```python
from build123d import *

# Parameters (mm, degrees)
SKETCH1_R           = 1.25
BOSS_EXTRUDE1_DEPTH = 0.1


with BuildPart() as part:
    # Sketch1 → Boss-Extrude1 (new body)
    with BuildSketch(Plane(origin=(0, 0, 0), x_dir=(1, 0, 0), z_dir=(0, 1, 0))):
        with BuildLine():
            Line((-34.25, 1.4), (-18.774596669, 1.4))
            ThreePointArc((-18.774596669, 1.4), (-18, 1.6), (-17.225403331, 1.4))
            Line((-17.225403331, 1.4), (17.225403331, 1.4))
            ThreePointArc((17.225403331, 1.4), (18, 1.6), (18.774596669, 1.4))
            Line((18.774596669, 1.4), (34.25, 1.4))
            Line((34.25, 1.4), (34.25, -1.4))
            Line((34.25, -1.4), (18.774596669, -1.4))
            ThreePointArc((18.774596669, -1.4), (18, -1.6), (17.225403331, -1.4))
            Line((17.225403331, -1.4), (-17.225403331, -1.4))
            ThreePointArc((-17.225403331, -1.4), (-18, -1.6), (-18.774596669, -1.4))
            Line((-18.774596669, -1.4), (-34.25, -1.4))
            Line((-34.25, -1.4), (-34.25, 1.4))
        make_face()
        with Locations(Location((-18, 0, 0), (0, 0, 270))):
            Circle(SKETCH1_R, mode=Mode.SUBTRACT)
        with Locations(Location((18, 0, 0), (0, 0, 90))):
            Circle(SKETCH1_R, mode=Mode.SUBTRACT)
    extrude(amount=BOSS_EXTRUDE1_DEPTH)


solid = part.part
```
Part model, mm, in its own coordinate system. Round coordinates to 2 decimals unless told otherwise and drop trailing zeros. Loops run counter-clockwise (first coordinate to the right, second up) from the corner with the lowest first, then second, coordinate; pieces in that order, holes last.
Item 1: Cut at B-B, the plane x = 18. Give the cut face in (y, z), then the cut area to 3 significant figures.
Item 2: Drill centre lines: line 1 (X direction, y = 0.05, z = 0); line 2 (Z direction, x = 18, y = 0.05); line 3 (Z direction, x = 25.5, y = 0.05). Where is each one in solid material? Low to high.
Item 3: Cut at A-A, the plane z = 0. Give the cut face in (x, y).
Item 4: Cut at C-C, the plane x = 7.5. Give the cut face in (y, z), then the cut area to 3 significant figures.
A:
1. outline: (0, -1.6) - (0.1, -1.6) - (0.1, -1.25) - (0, -1.25) - close; (0, 1.25) - (0.1, 1.25) - (0.1, 1.6) - (0, 1.6) - close
1. area: 0.0700 mm2
2. line 1: x = -34.25 to -19.25, -16.75 to 16.75, 19.25 to 34.25
2. line 2: z = -1.6 to -1.25, 1.25 to 1.6
2. line 3: z = -1.4 to 1.4
3. outline: (-34.25, 0) - (-19.25, 0) - (-19.25, 0.1) - (-34.25, 0.1) - close; (-16.75, 0) - (16.75, 0) - (16.75, 0.1) - (-16.75, 0.1) - close; (19.25, 0) - (34.25, 0) - (34.25, 0.1) - (19.25, 0.1) - close
4. outline: (0, -1.4) - (0.1, -1.4) - (0.1, 1.4) - (0, 1.4) - close
4. area: 0.280 mm2
